```python
from build123d import *

# Parameters (mm, degrees)
F1_DEPTH = 50.8
F4_DEPTH = 152.4


with BuildPart() as f1:
    # F0 (on Top) → F1 (new body)
    with BuildSketch(Plane.XY):
        with BuildLine():
            ThreePointArc((12.7, 0), (-8.9802561211, 8.9802561211), (0, -12.7))
            ThreePointArc((0, -12.7), (8.9802561211, -8.9802561211), (12.7, 0))
        make_face()
        with BuildLine():
            ThreePointArc((0, -11.1125), (-7.8577241059, 7.8577241059), (11.1125, 0))
            ThreePointArc((11.1125, 0), (7.8577241059, -7.8577241059), (0, -11.1125))
        make_face(mode=Mode.SUBTRACT)
    extrude(amount=F1_DEPTH)

    # F2 (on Front) → F3 (revolve)
    with BuildSketch(Plane.XZ):
        Polygon((11.1125, 51.7212620251), (11.1125, 50.8), (12.7, 50.8), (101.6, 101.6), (98.4002914561, 101.6), align=None)
    revolve(axis=Axis((0, 0, 76.2), (0, 0, 1)))

    # F0 (on Top) → F4 (cut)
    with BuildSketch(Plane.XY):
        with BuildLine():
            Line((72.9657332071, 61.2255198226), (10.9448599811, 9.1838279734))
            ThreePointArc((10.9448599811, 9.1838279734), (12.3733379566, 7.14375), (13.4258583195, 4.8866127978))
            Line((13.4258583195, 4.8866127978), (89.5057221299, 32.5774186518))
            ThreePointArc((89.5057221299, 32.5774186518), (82.4889197105, 47.625), (72.9657332071, 61.2255198226))
        make_face()
        with BuildLine():
            Line((93.8029384744, 16.5399889228), (14.0704407712, 2.4809983384))
            ThreePointArc((14.0704407712, 2.4809983384), (14.2875, 0), (14.0704407712, -2.4809983384))
            Line((14.0704407712, -2.4809983384), (93.8029384744, -16.5399889228))
            ThreePointArc((93.8029384744, -16.5399889228), (95.25, 0), (93.8029384744, 16.5399889228))
        make_face()
        with BuildLine():
            Line((32.5774186518, 89.5057221299), (4.8866127978, 13.4258583195))
            ThreePointArc((4.8866127978, 13.4258583195), (7.14375, 12.3733379566), (9.1838279734, 10.9448599811))
            Line((9.1838279734, 10.9448599811), (61.2255198226, 72.9657332071))
            ThreePointArc((61.2255198226, 72.9657332071), (47.625, 82.4889197105), (32.5774186518, 89.5057221299))
        make_face()
        with BuildLine():
            Line((0, -95.25), (0, -14.2875))
            ThreePointArc((0, -14.2875), (-1.2452376745, -14.233131749), (-2.4809983384, -14.0704407712))
            Line((-2.4809983384, -14.0704407712), (-16.5399889228, -93.8029384744))
            ThreePointArc((-16.5399889228, -93.8029384744), (-8.3015844967, -94.8875449932), (0, -95.25))
        make_face()
        with BuildLine():
            ThreePointArc((2.4809983384, -14.0704407712), (1.2452376745, -14.233131749), (0, -14.2875))
            Line((0, -14.2875), (0, -95.25))
            ThreePointArc((0, -95.25), (8.3015844967, -94.8875449932), (16.5399889228, -93.8029384744))
            Line((16.5399889228, -93.8029384744), (2.4809983384, -14.0704407712))
        make_face()
        with BuildLine():
            Line((61.2255198226, -72.9657332071), (9.1838279734, -10.9448599811))
            ThreePointArc((9.1838279734, -10.9448599811), (7.14375, -12.3733379566), (4.8866127978, -13.4258583195))
            Line((4.8866127978, -13.4258583195), (32.5774186518, -89.5057221299))
            ThreePointArc((32.5774186518, -89.5057221299), (47.625, -82.4889197105), (61.2255198226, -72.9657332071))
        make_face()
        with BuildLine():
            Line((89.5057221299, -32.5774186518), (13.4258583195, -4.8866127978))
            ThreePointArc((13.4258583195, -4.8866127978), (12.3733379566, -7.14375), (10.9448599811, -9.1838279734))
            Line((10.9448599811, -9.1838279734), (72.9657332071, -61.2255198226))
            ThreePointArc((72.9657332071, -61.2255198226), (82.4889197105, -47.625), (89.5057221299, -32.5774186518))
        make_face()
        with BuildLine():
            Line((-32.5774186518, -89.5057221299), (-4.8866127978, -13.4258583195))
            ThreePointArc((-4.8866127978, -13.4258583195), (-7.14375, -12.3733379566), (-9.1838279734, -10.9448599811))
            Line((-9.1838279734, -10.9448599811), (-61.2255198226, -72.9657332071))
            ThreePointArc((-61.2255198226, -72.9657332071), (-47.625, -82.4889197105), (-32.5774186518, -89.5057221299))
        make_face()
        with BuildLine():
            Line((-72.9657332071, -61.2255198226), (-10.9448599811, -9.1838279734))
            ThreePointArc((-10.9448599811, -9.1838279734), (-12.3733379566, -7.14375), (-13.4258583195, -4.8866127978))
            Line((-13.4258583195, -4.8866127978), (-89.5057221299, -32.5774186518))
            ThreePointArc((-89.5057221299, -32.5774186518), (-82.4889197105, -47.625), (-72.9657332071, -61.2255198226))
        make_face()
        with BuildLine():
            Line((-93.8029384744, -16.5399889228), (-14.0704407712, -2.4809983384))
            ThreePointArc((-14.0704407712, -2.4809983384), (-14.2875, 0), (-14.0704407712, 2.4809983384))
            Line((-14.0704407712, 2.4809983384), (-93.8029384744, 16.5399889228))
            ThreePointArc((-93.8029384744, 16.5399889228), (-95.25, 0), (-93.8029384744, -16.5399889228))
        make_face()
        with BuildLine():
            Line((-89.5057221299, 32.5774186518), (-13.4258583195, 4.8866127978))
            ThreePointArc((-13.4258583195, 4.8866127978), (-12.3733379566, 7.14375), (-10.9448599811, 9.1838279734))
            Line((-10.9448599811, 9.1838279734), (-72.9657332071, 61.2255198226))
            ThreePointArc((-72.9657332071, 61.2255198226), (-82.4889197105, 47.625), (-89.5057221299, 32.5774186518))
        make_face()
        with BuildLine():
            Line((-16.5399889228, 93.8029384744), (-2.4809983384, 14.0704407712))
            ThreePointArc((-2.4809983384, 14.0704407712), (0, 14.2875), (2.4809983384, 14.0704407712))
            Line((2.4809983384, 14.0704407712), (16.5399889228, 93.8029384744))
            ThreePointArc((16.5399889228, 93.8029384744), (0, 95.25), (-16.5399889228, 93.8029384744))
        make_face()
        with BuildLine():
            Line((-61.2255198226, 72.9657332071), (-9.1838279734, 10.9448599811))
            ThreePointArc((-9.1838279734, 10.9448599811), (-7.14375, 12.3733379566), (-4.8866127978, 13.4258583195))
            Line((-4.8866127978, 13.4258583195), (-32.5774186518, 89.5057221299))
            ThreePointArc((-32.5774186518, 89.5057221299), (-47.625, 82.4889197105), (-61.2255198226, 72.9657332071))
        make_face()
    extrude(amount=F4_DEPTH, mode=Mode.SUBTRACT)


solid = f1.part
```
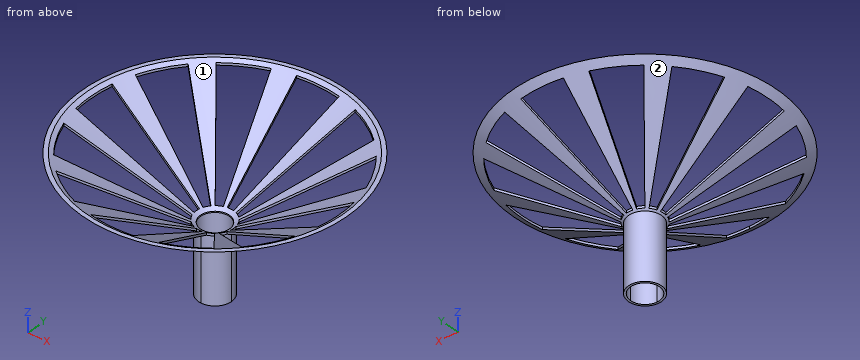
Input: part model. Units: mm. Frame: model coordinates. Face numbers are marked on the shaded views. Round coordinates to 2 decimals unless told otherwise and drop trailing zeros. Loops run counter-clockwise (first coordinate to the right, second up) from the corner with the lowest first, then second, coordinate; pieces in that order, holes last. Notation, with made-up numbers: (-24, 17) -> (-16, 17) arc R18 cw to (-16, 47) -> close; hole circle Ø11 at (78.25, -32). An arc over 180 degrees is marked (long way). Use one line per item in the form item = value. Start each with the question number.
Item 1: Material intervals for L1, parallel to X at y = 0, z = 51.4; L2, parallel to X at y = 0, z = 51.05; L3, parallel to Y at x = 0, z = 51, sorted ascending. Write a range as from..to.
Item 2: Section query A-A on z = 28.5. Return the cut outline in (x, y) (1 decimal), then the cut area to 3 significant figures.
Item 3: Mould query, pull axis X, two halves, no side actions, for the marked faces 1 and 2. Classes: pulls with the +X half, pulls with the -X half, needs draft (parallel to the pull), parting line crosses it, or undercut.
Item 4: Section query B-B on y = 40. Count the separate pieces of the cut face and the enclosed holes in it, then the cut area to 3 significant figures.
Item 5: Contact query for flat-ended pins moving along their axis: pin 1 Ø1 at (y, z) = (0.5, 24) entering from +X; pin 2 Ø1 at (x, y) = (14.5, 12.5) entering from +Z. Output: stop coordinate, or through.
Ans:
q1.L1 = -13.75..-11.11, 11.11..13.75
q1.L2 = -13.14..-11.11, 11.11..13.14
q1.L3 = -13.05..-11.11, 11.11..13.05
q2.outline = circle Ø25.4 at (0, 0); hole circle Ø22.2 at (0, 0)
q2.area = 119 mm^2
q3.face_1 = undercut
q3.face_2 = parting line crosses it
q4.separate_pieces = 6
q4.enclosed_holes = 0
q4.area = 98.1 mm^2
q5.pin_1 = 12.7
q5.pin_2 = 56.6
